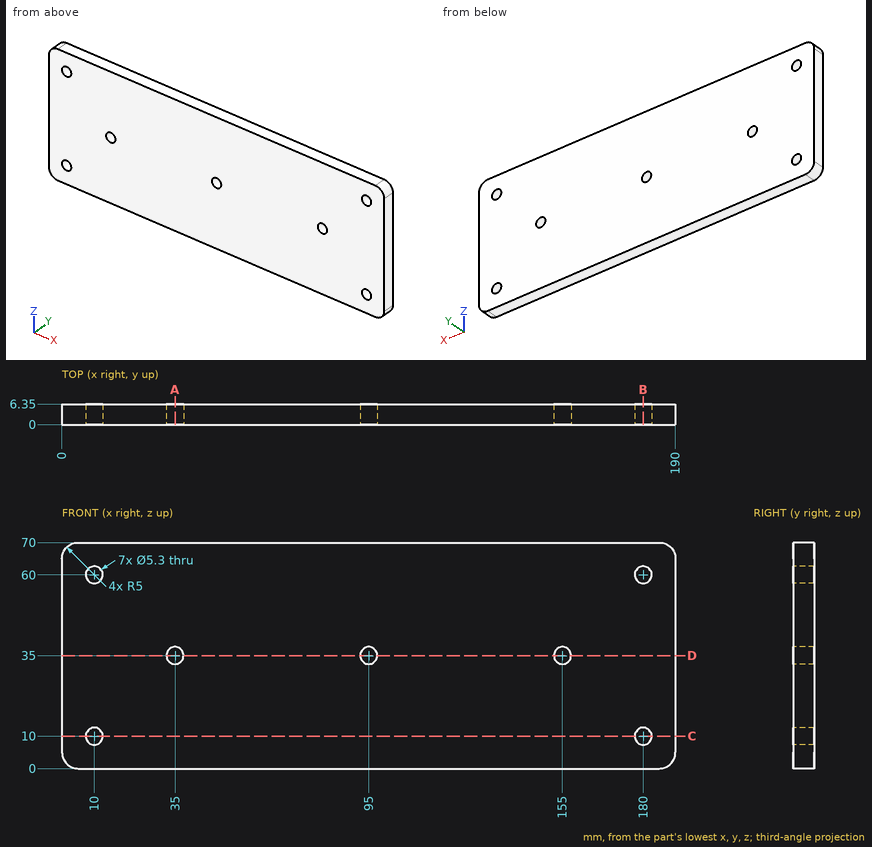
Could you check a few things on this drawing? It's one solid part, dimensions in mm from its lowest x, y, z. Coordinates: 2 decimals unless noted, no trailing zeros. Order: outer loops, then holes, each group sorted by start corner. A loop starts at its lowest first (then second) coordinate and runs counter-clockwise, first axis right, second up.
1. If we section it at A-A (x = 35): Please give me the cut outline in (y, z).
2. I need wall thicknesses on line 1 (X direction, y = 4.75, z = 35); line 2 (X direction, y = 3.5, z = 60); line 3 (Z direction, x = 180, y = 3.25). Which ranges of each line are inside material? Lowest first, please.
3. If we section it at C-C (z = 10): Please give me the cut outline in (x, y).
4. If we section it at B-B (x = 180): Please give me the cut outline in (y, z).
5. If we section it at D-D (z = 35): Please give me the cut outline in (x, y).
Entries:
1. outline: (0, 0) - (6.35, 0) - (6.35, 32.35) - (0, 32.35) - close; (0, 37.65) - (6.35, 37.65) - (6.35, 70) - (0, 70) - close
2. line 1: x = 0 to 32.35, 37.65 to 92.35, 97.65 to 152.35, 157.65 to 190
2. line 2: x = 0 to 7.35, 12.65 to 177.35, 182.65 to 190
2. line 3: z = 0 to 7.35, 12.65 to 57.35, 62.65 to 70
3. outline: (0, 0) - (7.35, 0) - (7.35, 6.35) - (0, 6.35) - close; (12.65, 0) - (177.35, 0) - (177.35, 6.35) - (12.65, 6.35) - close; (182.65, 0) - (190, 0) - (190, 6.35) - (182.65, 6.35) - close
4. outline: (0, 0) - (6.35, 0) - (6.35, 7.35) - (0, 7.35) - close; (0, 12.65) - (6.35, 12.65) - (6.35, 57.35) - (0, 57.35) - close; (0, 62.65) - (6.35, 62.65) - (6.35, 70) - (0, 70) - close
5. outline: (0, 0) - (32.35, 0) - (32.35, 6.35) - (0, 6.35) - close; (37.65, 0) - (92.35, 0) - (92.35, 6.35) - (37.65, 6.35) - close; (97.65, 0) - (152.35, 0) - (152.35, 6.35) - (97.65, 6.35) - close; (157.65, 0) - (190, 0) - (190, 6.35) - (157.65, 6.35) - close
